Design review of the part built by this model. Coordinates are the model's own, in mm. Face numbers are marked on the shaded views. A direction names the side the tool comes from. Coordinates: 2 decimals unless noted, no trailing zeros. Write each loop counter-clockwise with the first axis right and the second up, starting at its lowest first coordinate (ties: lowest second). Pieces come first, ordered by that corner, then holes. Notation, with made-up numbers: (19.5, 64.5) - (44.5, 64.5) arc R20 cw to (44.5, 82.5) - close; hole circle Ø2 at (-14, 75). An arc over 180 degrees is marked (long way). Answer as CSV lines item,"result". Start each with the question number.
Q1. We need section B-B (y = 12). Write out the cut boundary in (x, z).
Q2. We need section A-A (z = 0). Write out the cut boundary in (x, y), plus the area to 3 significant figures.
Q3. Clearance check with flat-ended pins moving along their axes: pin 1 (2 mm diameter, centred on x = -1.5, y = 4.5, fed in from -Z); pin 2 (1.5 mm diameter, centred on y = 2.5, z = 1.5, fed in from -X); pin 3 (8 mm diameter, centred on x = -6, y = 14, fed in from +Z). State where each tip first meets the part, or that it passes through.
Q4. For line 1 along Z through (x, y) = (5.75, 5.5); line 2 along X through (y, z) = (8.25, 3.5); line 3 along Z through (x, y) = (3.5, 9), list the stretches that pass through material, from the lowest coordinate up. Write a range as [from, to].
Q5. We need section C-C (y = 6.5). Write out the cut boundary in (x, z), plus the area to 3 significant figures.
Q6. Machinability: for the marked faces 1 and 2, which of the approach directions +Z, -Z, +X, -X, +Y, -Y give a long, thin tool a straight path to every point of the face, cutting with its end or side? Answer none if there is none.
Q7. Mouldability with a two-part tool opening along Z and no side actions: class the marked faces 3, 4 and 5 as pulls with the +Z half, pulls with the -Z half, needs draft (parallel to the pull), parting line crosses it, or undercut.
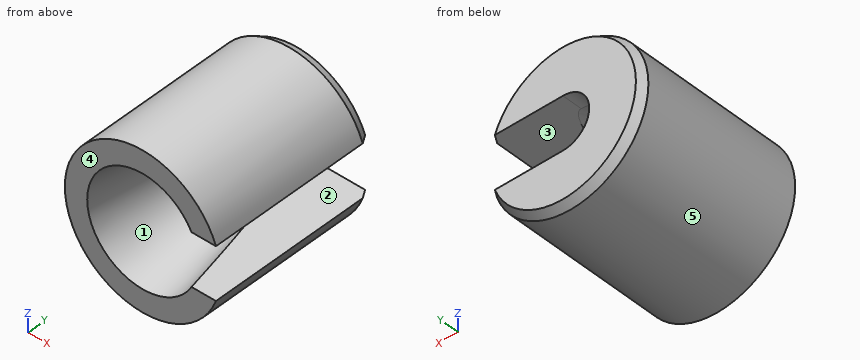
from build123d import *

# Parameters (mm, degrees)
SKETCH1_R           = 8
SKETCH1_R_2         = 2.7
BOSS_EXTRUDE1_DEPTH = 17.5
CHAMFER1_SIZE       = 3
CHAMFER1_SIZE2      = 15.433662048
CHAMFER2_SIZE       = 0.5
CHAMFER2_SIZE2      = 0.866025404
SKETCH2_W           = 11.3806618
SKETCH2_H           = 5.4
CUT_EXTRUDE1_DEPTH  = 20


with BuildPart() as part:
    # Sketch1 → Boss-Extrude1 (new body)
    with BuildSketch(Plane(origin=(0, 0, 0), x_dir=(1, 0, 0), z_dir=(0, 1, 0))):
        with Locations(Location((0, 0, 0), (0, 0, 270))):
            Circle(SKETCH1_R)
        with Locations(Location((0, 0, 0), (0, 0, 270))):
            Circle(SKETCH1_R_2, mode=Mode.SUBTRACT)
    extrude(amount=BOSS_EXTRUDE1_DEPTH)

    # Chamfer1
    chamfer1_edges = [part.edges().sort_by_distance(p)[0] for p in [
        (0, 0, -2.7),
    ]]
    chamfer1_side = [part.faces().sort_by_distance(p)[0] for p in [
        (0, 0, -7.77372583),
    ]]
    chamfer(chamfer1_edges, length=CHAMFER1_SIZE, length2=CHAMFER1_SIZE2, reference=chamfer1_side[0])

    # Chamfer2
    chamfer2_edges = [part.edges().sort_by_distance(p)[0] for p in [
        (0, 17.5, -8),
    ]]
    chamfer2_side = [part.faces().sort_by_distance(p)[0] for p in [
        (0, 17.5, -7.77372583),
    ]]
    chamfer(chamfer2_edges, length=CHAMFER2_SIZE, length2=CHAMFER2_SIZE2, reference=chamfer2_side[0])

    # Sketch2 → Cut-Extrude1 (cut)
    with BuildSketch(Plane(origin=(0, 17.5, 0), x_dir=(1, 0, 0), z_dir=(0, 1, 0))):
        with Locations((5.6903309, 0)):
            Rectangle(SKETCH2_W, SKETCH2_H)
    extrude(amount=-CUT_EXTRUDE1_DEPTH, mode=Mode.SUBTRACT)


solid = part.part
Results list:
1,outline,"(2.01, -2.7) arc R3.37 cw (long way) to (2.01, 2.7) - (7.53, 2.7) arc R8 ccw (long way) to (7.53, -2.7) - close"
2,outline,"(-8, 0) - (-5.7, 0) - (-2.7, 15.43) - (-2.7, 17.5) - (-7.5, 17.5) - (-8, 16.63) - close"
2,area,"69.4 mm2"
3,pin 1,"stops at z = -7.98"
3,pin 2,"stops at x = -7.96"
3,pin 3,"stops at z = 7.75"
4,line 1,"z = [-5.56, -2.7], [2.7, 5.56]"
4,line 2,"x = [-7.19, -2.13], [2.13, 7.19]"
4,line 3,"z = [-7.19, -2.7], [2.7, 7.19]"
5,outline,"(3.52, -2.7) arc R4.44 cw (long way) to (3.52, 2.7) - (7.53, 2.7) arc R8 ccw (long way) to (7.53, -2.7) - close"
5,area,"119 mm2"
6,face 1,"-Y"
6,face 2,"+X, +Y, -Y"
7,face 3,"undercut"
7,face 4,"needs draft"
7,face 5,"parting line crosses it"
